Design review of the part built by this model. Coordinates are the model's own, in mm. A direction names the side the tool comes from. Give positions to 0.01 mm unless a question says otherwise; leave off trailing zeros. Loops run counter-clockwise (first coordinate to the right, second up) from the corner with the lowest first, then second, coordinate; pieces in that order, holes last. Notation, with made-up numbers: M 88.5,12.25 L 101.5,12.25 A28 cw 101.5,36.25 Z; hole C -4,81 d10. An arc over 180 degrees is marked long. Answer as CSV lines item,"result".
```python
from build123d import *

# Parameters (mm, degrees)
PAD_DEPTH = 305


with BuildPart() as part:
    # Sketch → Pad (new body)
    with BuildSketch(Plane.XZ):
        with BuildLine():
            ThreePointArc((6, 5.262), (0, 11.262), (-6, 5.262))
            Line((-6, 0), (-6, 5.262))
            Line((-11, 0), (-6, 0))
            Line((-11, 1), (-11, 0))
            Line((-7, 1), (-11, 1))
            Line((-7, 1), (-7, 5.262))
            ThreePointArc((7, 5.262), (0, 12.262), (-7, 5.262))
            Line((7, 5.262), (7, 1))
            Line((11, 1), (7, 1))
            Line((11, 0), (11, 1))
            Line((6, 0), (11, 0))
            Line((6, 5.262), (6, 0))
        make_face()
    extrude(amount=PAD_DEPTH)


solid = part.part
```
1. The part is to be moulded in two halves that separate along X. For faces 3 (the cylindrical face through (0.13, -150.36, 11.26)), 4 (the cylindrical face through (0.15, -150.36, 12.26)), 5 (the flat face through (1.7, 0, 11.2)), say which applies: pulls with the +X half, pulls with the -X half, needs draft (parallel to the pull), parting line crosses it, or undercut.
Answer block:
face 3,"undercut"
face 4,"parting line crosses it"
face 5,"needs draft"
2. We need section A-A, the plane y = -57. Write out the cut boundary in (x, z), plus the area to 3 significant figures.
Answer block:
outline,"M -11,0 L -6,0 L -6,5.26 A6 cw 6,5.26 L 6,0 L 11,0 L 11,1 L 7,1 L 7,5.26 A7 ccw -7,5.26 L -7,1 L -11,1 Z"
area,"38.9 mm²"
3. We need section B-B, the plane x = 0. Write out the cut boundary in (y, z).
Answer block:
outline,"M -305,11.26 L 0,11.26 L 0,12.26 L -305,12.26 Z"
4. For faces 1 (the flat face through (-9, -150, 0)), 2 (the flat face through (-6, -150, 3)), list the 3-axis set-ups (+Z, -Z, +X, -X, +Y, -Y) from which the entire face can be reached by the end or side of a thin tool; tool diameter is ignored.
Answer block:
face 1,"-Z, +X, -X, +Y, -Y"
face 2,"-Z, +Y, -Y"
5. For P1, Ø3.5, axis at y = -113.5, z = 4, coming from the -X side; P2, Ø1, axis at y = -102.5, z = 7, coming from the -X side; P3, Ø4, axis at x = 3.5, y = -160.5, coming from the -Z side, all flat-tipped, find the tip position at first contact; note any pin that passes through.
Answer block:
P1,"x = -7"
P2,"x = -6.89"
P3,"z = 7.66"
6. To check wall thickness, follow L1, parallel to X at y = -53, z = 6; L2, parallel to Z at x = -7.25, y = -70; L3, parallel to Z at x = 0.5, y = -24. State the ranges of each line that lie inside material, in increasing order. Write a range as [from, to].
Answer block:
L1,"[-6.96, -5.95], [5.95, 6.96]"
L2,"[0, 1]"
L3,"[11.24, 12.24]"
